Source: CAD feature listing. Evaluate the final solid. Frame: model axes, mm. Round coordinates to 2 decimals unless told otherwise and drop trailing zeros. Write each loop counter-clockwise with the first axis right and the second up, starting at its lowest first coordinate (ties: lowest second). Pieces come first, ordered by that corner, then holes. Notation, with made-up numbers: M -32,27.5 L 20,27.5 A16 ccw 20,55.5 Z; hole C 17,-22.75 d1. An arc over 180 degrees is marked long. Answer in a Markdown table with one row per item.
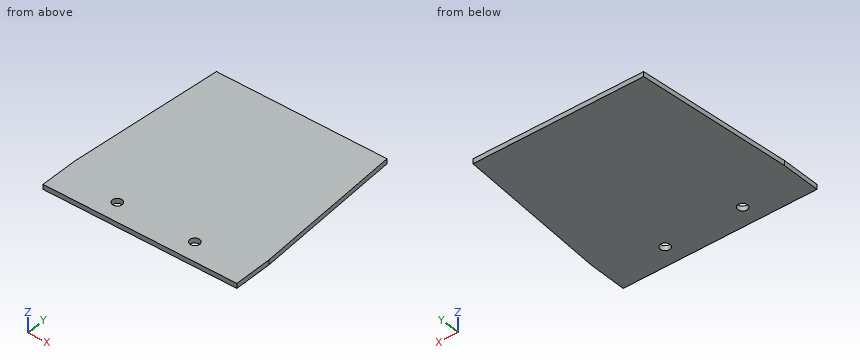
from build123d import *

# Parameters (mm, degrees)
SKETCH1_W           = 127
SKETCH1_H           = 25.4
BOSS_EXTRUDE1_DEPTH = 3.175
SKETCH2_R           = 3.175
CUT_EXTRUDE1_DEPTH  = 3.175


with BuildPart() as part:
    # Sketch1 → Boss-Extrude1 (new body)
    with BuildSketch(Plane.XY):
        Polygon((55.88, 25.4), (63.5, -76.2), (-63.5, -76.2), (-55.88, 25.4), align=None)
        with Locations((0, -88.9)):
            Rectangle(SKETCH1_W, SKETCH1_H)
    extrude(amount=BOSS_EXTRUDE1_DEPTH)

    # Sketch2 → Cut-Extrude1 (cut)
    with BuildSketch(Plane.XY.offset(3.175)):
        with Locations((-25.4, -88.9)):
            Circle(SKETCH2_R)
        with Locations((25.4, -88.9)):
            Circle(SKETCH2_R)
    extrude(amount=-CUT_EXTRUDE1_DEPTH, mode=Mode.SUBTRACT)


solid = part.part
Q1. Section A-A (y = -88.9). Return loops of the section in (x, z) (3 decimals).
Solutions:
| item | result |
|---|---|
| outline | M -63.5,0 L -28.575,0 L -28.575,3.175 L -63.5,3.175 Z; M -22.225,0 L 22.225,0 L 22.225,3.175 L -22.225,3.175 Z; M 28.575,0 L 63.5,0 L 63.5,3.175 L 28.575,3.175 Z |
Q2. Contact query for a flat-ended pin moving along its axis: pin 1 Ø1 at (y, z) = (4, 2.5) entering from +X. Output: stop coordinate, or through.
Solutions:
| item | result |
|---|---|
| pin 1 | stops at x = 57.52 |
Q3. Section B-B (x = -25.4). Return loops of the section in (y, z) (3 decimals).
Solutions:
| item | result |
|---|---|
| outline | M -101.6,0 L -92.075,0 L -92.075,3.175 L -101.6,3.175 Z; M -85.725,0 L 25.4,0 L 25.4,3.175 L -85.725,3.175 Z |
Q4. Section D-D (y = -5). Return loops of the section in (x, z) (3 decimals), and give its area (3 significant figures).
Solutions:
| item | result |
|---|---|
| outline | M -58.16,0 L 58.16,0 L 58.16,3.175 L -58.16,3.175 Z |
| area | 369 mm2 |
Q5. Material intervals for probe 1 along Y at (x, z) = (-25.4, 1.45) (3 decimals); probe 2 along X at (y, z) = (-86, 1.25); probe 3 along Y at (x, z) = (-26.5, 1.8), sorted ascending.
Solutions:
| item | result |
|---|---|
| probe 1 | y = -101.6 to -92.075, -85.725 to 25.4 |
| probe 2 | x = -63.5 to -26.69, -24.11 to 24.11, 26.69 to 63.5 |
| probe 3 | y = -101.6 to -91.88, -85.92 to 25.4 |
Q6. Section C-C (z = 2.6). Return loops of the section in (x, y) (3 decimals).
Solutions:
| item | result |
|---|---|
| outline | M -63.5,-101.6 L 63.5,-101.6 L 63.5,-76.2 L 55.88,25.4 L -55.88,25.4 L -63.5,-76.2 Z; hole C -25.4,-88.9 d6.35; hole C 25.4,-88.9 d6.35 |
